```python
from build123d import *

# Parameters (mm, degrees)
SKETCH_1_W          = 69
SKETCH_1_H          = 35
EXTRUDE_1_DEPTH     = 3
SKETCH_2_W          = 2.9
SKETCH_2_H          = 16
SKETCH_2_W_2        = 6.9
EXTRUDE_2_DEPTH     = 17
CUT_EXTRUDE_1_REACH = 60.323
SKETCH_3_R          = 2.8
FILLET_1_R          = 10
FILLET_2_R          = 4
CUT_EXTRUDE_2_DEPTH = 10
FILLET_3_R          = 1.5
EXTRUDE_START       = -6.9
SKETCH_6_R          = 5.094551448
SKETCH_6_R_2        = 2.8
EXTRUDE_4_DEPTH     = 3
SKETCH_7_R          = 1.75
CUT_EXTRUDE_3_DEPTH = 10


with BuildPart() as part:
    # Эскиз1 → Бобышка-Вытянуть1 (new body)
    with BuildSketch(Plane.XY):
        with Locations((34.5, 17.5)):
            Rectangle(SKETCH_1_W, SKETCH_1_H)
    extrude(amount=EXTRUDE_1_DEPTH)

    # Эскиз2 → Бобышка-Вытянуть2 (add)
    with BuildSketch(Plane.XY.offset(3)):
        with Locations((34.5, 17.5)):
            Rectangle(SKETCH_2_W, SKETCH_2_H)
        with Locations((28.3, 17.5)):
            Rectangle(SKETCH_2_W, SKETCH_2_H)
        with Locations((42.7, 17.5)):
            Rectangle(SKETCH_2_W_2, SKETCH_2_H)
    extrude(amount=EXTRUDE_2_DEPTH)

    # Вырез-Вытянуть1: up to this face of the body (flat: up to its plane)
    cut_extrude_1_end = Plane(part.part.faces().sort_by_distance((35.95, 17.5, 11.5))[0])
    # Эскиз3 → Вырез-Вытянуть1 (cut, up to the picked face)
    with BuildSketch(Plane.ZY.offset(-26.85), mode=Mode.PRIVATE) as cut_extrude_1_sk1:
        with Locations((14, 17.5)):
            Circle(SKETCH_3_R)
    cut_extrude_1_tool1 = split(extrude(cut_extrude_1_sk1.sketch, amount=-CUT_EXTRUDE_1_REACH, mode=Mode.PRIVATE), bisect_by=cut_extrude_1_end, keep=Keep.BOTH, mode=Mode.PRIVATE)
    add(cut_extrude_1_tool1.solids().sort_by(Axis((26.85, 17.5, 14), (1, 0, 0)))[0], mode=Mode.SUBTRACT)

    # Скругление1
    # the kernel refuses this fillet: 10 mm, written as the material it takes off along each edge
    with BuildSketch(Plane(origin=(1.85, 25.5, 20), x_dir=(0, 0, -1), z_dir=(1, 0, 0)), Plane(origin=(54.75, 9.5, 20), x_dir=(0, 0, -1), z_dir=(-1, 0, 0))) as fillet_1_piece_1:
        with BuildLine():
            CenterArc((FILLET_1_R, -FILLET_1_R), FILLET_1_R, 90, 90)
            Line((0, -FILLET_1_R), (0, 0))
            Line((0, 0), (FILLET_1_R, 0))
        make_face()
    extrude(amount=52.9, mode=Mode.SUBTRACT)
    with BuildSketch(Plane(origin=(60.95, 25.5, 20), x_dir=(0, 0, -1), z_dir=(-1, 0, 0)), Plane(origin=(8.05, 9.5, 20), x_dir=(0, 0, -1), z_dir=(1, 0, 0))) as fillet_1_piece_2:
        with BuildLine():
            CenterArc((FILLET_1_R, FILLET_1_R), FILLET_1_R, 180, 90)
            Line((0, FILLET_1_R), (0, 0))
            Line((0, 0), (FILLET_1_R, 0))
        make_face()
    extrude(amount=52.9, mode=Mode.SUBTRACT)
    with BuildSketch(Plane(origin=(14.25, 25.5, 20), x_dir=(0, 0, -1), z_dir=(1, 0, 0)), Plane(origin=(71.15, 9.5, 20), x_dir=(0, 0, -1), z_dir=(-1, 0, 0))) as fillet_1_piece_3:
        with BuildLine():
            CenterArc((FILLET_1_R, -FILLET_1_R), FILLET_1_R, 90, 90)
            Line((0, -FILLET_1_R), (0, 0))
            Line((0, 0), (FILLET_1_R, 0))
        make_face()
    extrude(amount=56.9, mode=Mode.SUBTRACT)

    # Скругление2
    fillet_2_edges = [part.edges().sort_by_distance(p)[0] for p in [
        (46.15, 17.5, 3),
        (26.85, 17.5, 3),
    ]]
    fillet(fillet_2_edges, radius=FILLET_2_R)

    # Эскиз4 → Вырез-Вытянуть2 (cut)
    with BuildSketch(Plane.ZY.offset(-39.25)):
        Polygon((14.008077291, 22.292000427), (9.854044541, 19.902995352), (9.84596725, 15.110994925), (13.991922709, 12.707999573), (18.145955459, 15.097004648), (18.15403275, 19.889005075), align=None)
    extrude(amount=-CUT_EXTRUDE_2_DEPTH, mode=Mode.SUBTRACT)

    # Скругление3
    fillet_3_edges = [part.edges().sort_by_distance(p)[0] for p in [
        (34.5, 25.5, 3),
        (33.05, 17.5, 3),
        (34.5, 9.5, 3),
        (35.95, 17.5, 3),
        (39.25, 17.5, 3),
        (44.7, 9.5, 3),
        (44.7, 25.5, 3),
        (29.75, 17.5, 3),
        (26.3, 25.5, 3),
        (26.3, 9.5, 3),
    ]]
    fillet(fillet_3_edges, radius=FILLET_3_R)

    # Эскиз6 → Бобышка-Вытянуть4 (add)
    with BuildSketch(Plane(origin=(46.15, 0, 0), x_dir=(0, 0, -1), z_dir=(1, 0, 0)).offset(EXTRUDE_START)):
        with Locations((-14, 17.5)):
            Circle(SKETCH_6_R)
        with Locations(Location((-14, 17.5, 0), (0, 0, 180))):
            Circle(SKETCH_6_R_2, mode=Mode.SUBTRACT)
    extrude(amount=EXTRUDE_4_DEPTH)

    # Эскиз7 → Вырез-Вытянуть3 (cut)
    with BuildSketch(Plane.XY.offset(3)):
        with Locations((7, 17.5)):
            Circle(SKETCH_7_R)
        with Locations((62, 17.5)):
            Circle(SKETCH_7_R)
    extrude(amount=-CUT_EXTRUDE_3_DEPTH, mode=Mode.SUBTRACT)


solid = part.part
```
The model under review builds one solid part; all positions refer to its coordinate system, in mm. A direction names the side the tool comes from. Give positions to 0.01 mm unless a question says otherwise; leave off trailing zeros. Write each loop counter-clockwise with the first axis right and the second up, starting at its lowest first coordinate (ties: lowest second). Pieces come first, ordered by that corner, then holes. Notation, with made-up numbers: M 10.25,-26.5 L 66.25,-26.5 A19 ccw 66.25,-15.5 Z; hole C 13.25,-2.5 d4. An arc over 180 degrees is marked long. Write item = value, one per line. Start each with the question number.
Q1. We need section A-A (x = 7). State the section outline as (y, z) points.
Q2. We need section C-C (y = 24). State the section outline as (x, z) points.
Q3. We need section B-B (z = 15). State the section outline as (x, y) points.
Q4. Mouldability with a two-part tool opening along Z and no side actions: class faces 1 (the face through (35.95, 17, 10)), 2 (the face through (38.8, 17.63, 3.43)), 3 (the face through (42.25, 15, 16)) as released by +Z, released by -Z, zero draft, split by the parting line, or undercut.
Q5. For line 1 (X direction, y = 25, z = 7.25); line 2 (X direction, y = 20, z = 10.5); line 3 (Y direction, x = 7, z = 2), list the stretches that pass through material, from the lowest coordinate up.
Q6. Machinability: for faces 4 (the face through (32.6, 17.63, 3.43)), 5 (the face through (34.48, 23.306, 16.25)), 6 (the face through (28, 9.5, 7)), which of the approach directions +Z, -Z, +X, -X, +Y, -Y give a long, thin tool a straight path to every point of the face, cutting with its end or side? Answer none if there is none.
Q7. We need section D-D (z = 6). State the section outline as (x, y) points.
Q8. Clearance check with flat-ended pins moving along their axes: pin 1 (1.5 mm diameter, centred on x = 48.5, y = 22.5, fed in from +Z); pin 2 (2.5 mm diameter, centred on x = 34, z = 8, fed in from -Y); pin 3 (10 mm diameter, centred on x = 10, z = 7, fed in from -Y); pin 4 (1.9 mm diameter, centred on x = 27.5, z = 6.5, fed in from +Y). State where each tip first meets the part, or that it passes through.
Result set:
q1.outline = M 0,0 L 15.75,0 L 15.75,3 L 0,3 Z; M 19.25,0 L 35,0 L 35,3 L 19.25,3 Z
q2.outline = M 0,0 L 69,0 L 69,3 L 50.15,3 A4 cw 46.15,7 L 46.15,15.27 L 39.25,15.27 L 39.25,4.5 A1.5 cw 37.75,3 L 37.45,3 A1.5 cw 35.95,4.5 L 35.95,15.27 L 33.05,15.27 L 33.05,4.5 A1.5 cw 31.55,3 L 31.25,3 A1.5 cw 29.75,4.5 L 29.75,15.27 L 26.85,15.27 L 26.85,7 A4 cw 22.85,3 L 0,3 Z
q3.outline = M 26.85,10.84 L 29.75,10.84 L 29.75,14.88 L 26.85,14.88 Z; M 26.85,20.12 L 29.75,20.12 L 29.75,24.16 L 26.85,24.16 Z; M 33.05,10.84 L 35.95,10.84 L 35.95,14.88 L 33.05,14.88 Z; M 33.05,20.12 L 35.95,20.12 L 35.95,24.16 L 33.05,24.16 Z; M 39.25,10.84 L 46.15,10.84 L 46.15,13.29 L 42.25,13.29 L 42.25,14.88 L 39.25,14.88 Z; M 39.25,20.12 L 42.25,20.12 L 42.25,21.72 L 46.15,21.72 L 46.15,24.16 L 39.25,24.16 Z
q4.face_1 = zero draft
q4.face_2 = released by +Z
q4.face_3 = undercut
q5.line_1 = 26.85 to 29.75, 33.05 to 35.95, 39.25 to 46.15
q5.line_2 = 26.85 to 29.75, 33.05 to 35.95, 39.25 to 42.25
q5.line_3 = 0 to 15.75, 19.25 to 35
q6.face_4 = +Z, +Y, -Y
q6.face_5 = +Z, +X, -X, +Y
q6.face_6 = +Z, +X, -X, -Y
q7.outline = M 26.72,9.5 L 29.75,9.5 L 29.75,25.5 L 26.72,25.5 Z; M 33.05,9.5 L 35.95,9.5 L 35.95,25.5 L 33.05,25.5 Z; M 39.25,9.5 L 46.28,9.5 L 46.28,25.5 L 39.25,25.5 Z
q8.pin_1 = 3.8
q8.pin_2 = 9.5
q8.pin_3 = 0
q8.pin_4 = 25.5
